Here's how the part is built. I have some questions about the finished solid (model axes, mm). Coordinates: 2 decimals unless noted, no trailing zeros. Write each loop counter-clockwise with the first axis right and the second up, starting at its lowest first coordinate (ties: lowest second). Pieces come first, ordered by that corner, then holes. Notation, with made-up numbers: (38.25, 24) -> (64.25, 24) arc R18 ccw to (64.25, 56) -> close; hole circle Ø9 at (47, -35). An arc over 180 degrees is marked (long way). Put each result on its own line as item: value. Start each with the question number.
Item 1: If we mould it in two halves opening along Z, with no side actions, what happens to faces 1 (the face through (88, 4.966, 99)), 2 (the face through (19.527, 0.008, 148.724)), 3 (the face through (-123.997, -0.076, -39.048))? For each: released by +Z, released by -Z, zero draft, split by the parting line, or undercut.
Item 2: I want a section at B-B, the plane y = -0.5. State how many separate pieces and enclosed holes the cut face has, then the cut area to 3 significant figures.
Item 3: For pin 1 (1.5 mm diameter, centred on y = 3.5, z = -35.5, fed in from +X); pin 2 (2.5 mm diameter, centred on x = -41.94, z = 132.23, fed in from -Y); pin 3 (4 mm diameter, centred on x = -6.5, y = -4, fed in from +Z), each with a flat end and sliding along its axis, tell me the tip position at first contact or that it passes through.
Item 4: I want a section at A-A, the plane x = 0. List the corners of the cut face in (y, z) for me, then the cut area to 3 significant figures.
Item 5: I need wall thicknesses on line 1 (Z direction, x = 0, y = 1.25); line 2 (X direction, y = 1.25, z = -131.5); line 3 (X direction, y = 3.5, z = 58). Which ranges of each line are inside material? Lowest first, please. Write a range as [from, to].
Autodesk Inventor part; units mm, degrees
ref_plane "YZ Plane" through (0, 0, 0) normal (1, 0, 0) x (0, 1, 0)
ref_plane "XZ Plane" through (0, 0, 0) normal (0, 1, 0) x (-1, 0, 0)
ref_plane "XY Plane" through (0, 0, 0) normal (0, 0, 1) x (1, 0, 0)
sketch "Boceto1" plane through (0, 0, 0) normal (0, 0, 1) x (1, 0, 0)
  line L0 (-150, 4.9659) -> (-130, 4.9659)
  line L1 (-130, 4.9659) -> (-130, -5.0341)
  line L2 (-130, -5.0341) -> (-150, -5.0341)
  line L3 (-150, -5.0341) -> (-150, 4.9659)
  line L4 (0, 0) -> (0, 54.3262)
  dimension "d0" = 20
  dimension "d1" = 10
  dimension "d2" = 150
revolve "Revolución1" add sketch "Boceto1" angle 360 about axis through (0, 0, 0) along (0, 1, 0)
chamfer "Chaflán1" distance 2 angle 45 4 edges at (150, 4.9659, 0) (130, 4.9659, 0) (150, -5.0341, 0) (130, -5.0341, 0)
sketch "Boceto2" plane through (0, 4.9659, 0) normal (0, 1, 0) x (1, 0, 0)
  point P0 (0, 0)
  point P1 (-138.7138, -0.9769)
hole "Agujero1" at (-138.7138, 4.9659, 0.9769) direction (0, -1, 0) diameter 4.134 end through all
pattern_circular "Patrón circular1" count 10 over 360 about axis through (0, -10, 0) along (0, 1, 0) of "Agujero1"
equation "\"d12\" = Grosor"
equation "\"Radio_pliegue\" = Grosor"
equation "\"Anchura_desahogo_plegado\" = Grosor"
equation "\"Profundidad_desahogo_plegado\" = 0.5 * Grosor"
equation "\"Tamaño_destalonado\" = 4 * Grosor"
equation "\"Remanente_mínimo\" = 2 * Grosor"
equation "\"Radiodetransición\" = Radio_pliegue"
equation "\"Tamaño_de_radio_de_Jacobi\" = Radio_pliegue"
equation "\"TamañoSeparación\" = Grosor"
Calculated:
1. face 1: zero draft
1. face 2: split by the parting line
1. face 3: undercut
2. separate pieces: 1
2. enclosed holes: 11
2. area: 17,500 mm2
3. pin 1: stops at x = 145.87
3. pin 2: passes through
3. pin 3: stops at z = 149.92
4. outline: (-5.03, -148) -> (-3.03, -150) -> (2.97, -150) -> (4.97, -148) -> (4.97, -132) -> (2.97, -130) -> (-3.03, -130) -> (-5.03, -132) -> close; (-5.03, 132) -> (-3.03, 130) -> (2.97, 130) -> (4.97, 132) -> (4.97, 148) -> (2.97, 150) -> (-3.03, 150) -> (-5.03, 148) -> close
4. area: 384 mm2
5. line 1: z = [-150, -130], [130, 150]
5. line 2: x = [-72.16, -45.86], [-41.73, 40], [43.87, 72.16]
5. line 3: x = [-137.75, -116.94], [116.94, 137.75]
